Autodesk Inventor part; units mm, degrees
ref_plane "YZ Plane" through (0, 0, 0) normal (1, 0, 0) x (0, 1, 0)
ref_plane "XZ Plane" through (0, 0, 0) normal (0, 1, 0) x (-1, 0, 0)
ref_plane "XY Plane" through (0, 0, 0) normal (0, 0, 1) x (1, 0, 0)
sketch "Sketch1" plane through (0, 0, 0) normal (0, 0, 1) x (1, 0, 0)
  line L0 (8, 0) -> (57, 0)
  line L1 (65, 8) -> (65, 87)
  line L2 (57, 95) -> (8, 95)
  line L3 (0, 87) -> (0, 8)
  arc A0 (0, 8) -> (8, 0) centre (8, 8) ccw
  arc A1 (8, 95) -> (0, 87) centre (8, 87) ccw
  arc A2 (65, 87) -> (57, 95) centre (57, 87) ccw
  arc A3 (57, 0) -> (65, 8) centre (57, 8) ccw
  point P0 (0, 0)
  point P1 (65, 95)
  point P2 (65, 0)
  point P3 (0, 95)
  dimension "d0" = 65
  dimension "d1" = 95
  dimension "d2" = 8
extrude "Extrusion1" add sketch "Sketch1" along normal blind 32
sketch "Sketch2" plane through (0, 0, 0) normal (0, 0, -1) x (-1, 0, 0)
  line L0 (-8, 12) -> (-57, 12) construction
  line L1 (-57, 12) -> (-57, 70) construction
  line L2 (-57, 70) -> (-8, 70) construction
  line L3 (-8, 70) -> (-8, 12) construction
  line L4 (-8, 0) -> (-57, 0)
  line L5 (-32.5, 0) -> (-32.5, 94.8442) construction
  circle A0 centre (-57, 12) radius 1.5
  circle A1 centre (-57, 70) radius 1.5
  circle A2 centre (-8, 70) radius 1.5
  circle A3 centre (-8, 12) radius 1.5
  line L6 (-16.9436, 109.56) -> (-16.9436, 104.8114)
  line L7 (-40.3748, 104.8114) -> (-28.4573, 104.8114)
  line L8 (0.0184, 88.6231) -> (0.0184, 5.8494)
  line L9 (-28.0001, -10.2773) -> (-40.3748, -10.2773)
  line L10 (-16.9436, -10.2773) -> (-16.9436, -14.3057)
  line L11 (-21.9436, -19.3057) -> (-23.0001, -19.3057)
  line L12 (-28.0001, -14.3057) -> (-28.0001, -10.2773)
  line L13 (-40.3748, -10.2773) -> (-40.3748, -14.3057)
  line L14 (-45.3748, -19.3057) -> (-47.2671, -19.3057)
  line L15 (-52.2671, -14.3057) -> (-52.2671, -10.2773)
  line L16 (-64.9916, 6.3782) -> (-64.9916, 88.5882)
  line L17 (-52.2671, 104.8114) -> (-52.2671, 109.56)
  line L18 (-47.2671, 114.56) -> (-45.3748, 114.56)
  line L19 (-40.3748, 109.56) -> (-40.3748, 104.8114)
  line L20 (-28.4573, 104.8114) -> (-28.4573, 109.56)
  line L21 (-23.4573, 114.56) -> (-21.9436, 114.56)
  line L22 (-15.7324, 83.4806) -> (-23.5066, 91.204)
  arc A4 (-23.5066, 91.204) -> (-27.0305, 92.6569) centre (-27.0305, 87.6569) ccw
  line L23 (-27.0305, 92.6569) -> (-42.3584, 92.6569)
  arc A5 (-42.3584, 92.6569) -> (-45.8878, 91.1985) centre (-42.3584, 87.6569) ccw
  line L24 (-45.8878, 91.1985) -> (-50.0687, 87.0321)
  arc A6 (-50.0687, 87.0321) -> (-51.5393, 83.4904) centre (-46.5393, 83.4904) ccw
  line L25 (-51.5393, 83.4904) -> (-51.5393, 49.6697)
  arc A7 (-51.5393, 49.6697) -> (-49.6635, 45.7659) centre (-46.5393, 49.6697) ccw
  line L26 (-49.6635, 45.7659) -> (-44.7373, 41.8235)
  arc A8 (-44.7373, 41.8235) -> (-41.6131, 40.7274) centre (-41.6131, 45.7274) ccw
  line L27 (-41.6131, 40.7274) -> (-23.3988, 40.7274)
  arc A9 (-23.3988, 40.7274) -> (-20.0405, 42.0231) centre (-23.3988, 45.7274) ccw
  line L28 (-20.0405, 42.0231) -> (-15.898, 45.7787)
  arc A10 (-15.898, 45.7787) -> (-14.2563, 49.483) centre (-19.2563, 49.483) ccw
  line L29 (-14.2563, 49.483) -> (-14.2563, 79.9335)
  arc A11 (-14.2563, 79.9335) -> (-15.7324, 83.4806) centre (-19.2563, 79.9335) ccw
  line L30 (-14.2563, 9.4113) -> (-14.2563, 25.1215)
  arc A12 (-14.2563, 25.1215) -> (-16.1322, 29.0254) centre (-19.2563, 25.1215) ccw
  line L31 (-16.1322, 29.0254) -> (-19.9618, 32.0901)
  arc A13 (-19.9618, 32.0901) -> (-23.0859, 33.1863) centre (-23.0859, 28.1863) ccw
  line L32 (-23.0859, 33.1863) -> (-41.6879, 33.1863)
  arc A14 (-41.6879, 33.1863) -> (-44.5033, 32.3183) centre (-41.6879, 28.1863) ccw
  line L33 (-44.5033, 32.3183) -> (-49.3548, 29.0127)
  arc A15 (-49.3548, 29.0127) -> (-51.5393, 24.8807) centre (-46.5393, 24.8807) ccw
  line L34 (-51.5393, 24.8807) -> (-51.5393, 7.149)
  arc A16 (-51.5393, 7.149) -> (-50.9681, 4.8281) centre (-46.5393, 7.149) ccw
  line L35 (-50.9681, 4.8281) -> (-49.1556, 1.3694)
  arc A17 (-49.1556, 1.3694) -> (-44.7268, -1.3097) centre (-44.7268, 3.6903) ccw
  line L36 (-44.7268, -1.3097) -> (-23.7592, -1.3097)
  arc A18 (-23.7592, -1.3097) -> (-19.8301, 0.5979) centre (-23.7592, 3.6903) ccw
  line L37 (-19.8301, 0.5979) -> (-15.3273, 6.3189)
  arc A19 (-15.3273, 6.3189) -> (-14.2563, 9.4113) centre (-19.2563, 9.4113) ccw
  arc A20 (-64.9916, 6.3782) -> (-63.7832, 3.1188) centre (-59.9916, 6.3782) ccw
  arc A21 (-63.7296, 91.909) -> (-64.9916, 88.5882) centre (-59.9916, 88.5882) ccw
  line L38 (-63.7296, 91.909) -> (-52.2671, 104.8114)
  arc A22 (-47.2671, 114.56) -> (-52.2671, 109.56) centre (-47.2671, 109.56) ccw
  arc A23 (-40.3748, 109.56) -> (-45.3748, 114.56) centre (-45.3748, 109.56) ccw
  arc A24 (-23.4573, 114.56) -> (-28.4573, 109.56) centre (-23.4573, 109.56) ccw
  arc A25 (-16.9436, 109.56) -> (-21.9436, 114.56) centre (-21.9436, 109.56) ccw
  line L39 (-16.9436, 104.8114) -> (-1.8245, 92.5003)
  arc A26 (0.0184, 88.6231) -> (-1.8245, 92.5003) centre (-4.9816, 88.6231) ccw
  arc A27 (-1.834, 1.9645) -> (0.0184, 5.8494) centre (-4.9816, 5.8494) ccw
  line L40 (-1.834, 1.9645) -> (-16.9436, -10.2773)
  arc A28 (-21.9436, -19.3057) -> (-16.9436, -14.3057) centre (-21.9436, -14.3057) ccw
  arc A29 (-28.0001, -14.3057) -> (-23.0001, -19.3057) centre (-23.0001, -14.3057) ccw
  arc A30 (-45.3748, -19.3057) -> (-40.3748, -14.3057) centre (-45.3748, -14.3057) ccw
  arc A31 (-52.2671, -14.3057) -> (-47.2671, -19.3057) centre (-47.2671, -14.3057) ccw
  line L41 (-52.2671, -10.2773) -> (-63.7832, 3.1188)
  circle A32 centre (-57, 70) radius 2
  circle A33 centre (-57, 12) radius 2
  circle A34 centre (-8, 70) radius 2
  circle A35 centre (-8, 12) radius 2
  circle A36 centre (-22.639, 109.6569) radius 1.75
  circle A37 centre (-46.639, -14.5983) radius 1.75
  circle A38 centre (-46.639, 109.6569) radius 1.75
  circle A39 centre (-22.639, -14.5983) radius 1.75
  point P0 (0, 0)
  dimension "d5" = 49
  dimension "d6" = 58
  dimension "d7" = 24.5
  dimension "d8" = 12
  dimension "d9" = 3
  dimension "d10" = 3
  dimension "d11" = 3
  dimension "d12" = 3
extrude "Extrusion2" cut sketch "Sketch2" against normal blind 10 contours A0 | A1 | A2 | A3
properties part number "RPI"
Design review of the part built by this model. Coordinates are the model's own, in mm. A direction names the side the tool comes from. Round coordinates to 2 decimals unless told otherwise and drop trailing zeros. Loops run counter-clockwise (first coordinate to the right, second up) from the corner with the lowest first, then second, coordinate; pieces in that order, holes last. Notation, with made-up numbers: (14, 41) - (52, 41) arc R33 ccw to (52, 78) - close; hole circle Ø5 at (69.5, -27.75). An arc over 180 degrees is marked (long way). One line per item, written item: value. Start each with the question number.
1) For faces 1 (the flat face through (32, 48, 0)), 2 (the flat face through (57, 70, 10)), list the 3-axis set-ups (+Z, -Z, +X, -X, +Y, -Y) from which the entire face can be reached by the end or side of a thin tool; tool diameter is ignored.
2) Consider section A-A on y = 70. Give the boundary of the cut face in (x, z), then the cut area to 3 significant figures.
3) To check wall thickness, follow L1, parallel to Y at x = 57, z = 3.25; L2, parallel to X at y = 70, z = 2.5; L3, parallel to Y at x = 4, z = 9.5. State the ranges of each line that lie inside material, in increasing order. Write a range as from..to.
4) Insertion check: pin 1 Ø0.9 at (x, y) = (56.5, 70.5) entering from -Z. The pin has a flat end and moves straight along its axis. Give the tip position at first contact, or say it passes through.
5) Draft analysis for pull direction Y (two halves, no side actions). For faces 3 (the cylindrical face through (2.406, 2.281, 15.776)), 4 (the cylindrical face through (55.57, 70.45, 4.93)), 5 (the cylindrical face through (9.5, 12.07, 4.93)), 6 (the flat face through (0, 48, 16)), state which applies: +Y half, -Y half, draft (parallel to the pull), parting line (faces both ways), or undercut.
Reported:
1. face 1: -Z, +X, -X, +Y, -Y
1. face 2: -Z
2. outline: (0, 0) - (6.5, 0) - (6.5, 10) - (9.5, 10) - (9.5, 0) - (55.5, 0) - (55.5, 10) - (58.5, 10) - (58.5, 0) - (65, 0) - (65, 32) - (0, 32) - close
2. area: 2,020 mm^2
3. L1: y = 0..10.5, 13.5..68.5, 71.5..95
3. L2: x = 0..6.5, 9.5..55.5, 58.5..65
3. L3: y = 1.07..93.93
4. pin 1: stops at z = 10
5. face 3: -Y half
5. face 4: undercut
5. face 5: undercut
5. face 6: draft
